```python
from build123d import *

# Parameters (mm, degrees)
SKETCH_1_W          = 15
SKETCH_1_H          = 15
SKETCH_1_W_2        = 13
SKETCH_1_H_2        = 13
EXTRUDE_1_DEPTH     = 155
SKETCH_2_R          = 1.6
CUT_EXTRUDE_1_DEPTH = 157.444878472
SKETCH_3_R          = 1.6
CUT_EXTRUDE_2_DEPTH = 157.444878472


with BuildPart() as part:
    # 草图1 → 拉伸-薄壁1 (new body)
    with BuildSketch(Plane.XY):
        with Locations((7.5, -7.5)):
            Rectangle(SKETCH_1_W, SKETCH_1_H)
        with Locations((7.5, -7.5)):
            Rectangle(SKETCH_1_W_2, SKETCH_1_H_2, mode=Mode.SUBTRACT)
    extrude(amount=EXTRUDE_1_DEPTH)

    # 草图2 → 切除-拉伸1 (cut, through all)
    with BuildSketch(Plane(origin=(15, 0, 0), x_dir=(0, 0, -1), z_dir=(1, 0, 0))):
        with Locations((-130, -3.75)):
            Circle(SKETCH_2_R)
        with Locations((-130, -11.25)):
            Circle(SKETCH_2_R)
        with Locations((-120, -11.25)):
            Circle(SKETCH_2_R)
        with Locations((-120, -3.75)):
            Circle(SKETCH_2_R)
        with Locations((-20, -3.75)):
            Circle(SKETCH_2_R)
        with Locations((-20, -11.25)):
            Circle(SKETCH_2_R)
        with Locations((-30, -11.25)):
            Circle(SKETCH_2_R)
        with Locations((-30, -3.75)):
            Circle(SKETCH_2_R)
        Polygon((-105, -1), (-110.629165125, -4.25), (-110.629165125, -10.75), (-105, -14), (-99.370834875, -10.75), (-99.370834875, -4.25), align=None)
        Polygon((-84.370834875, -10.75), (-84.370834875, -4.25), (-90, -1), (-95.629165125, -4.25), (-95.629165125, -10.75), (-90, -14), align=None)
        Polygon((-69.370834875, -10.75), (-69.370834875, -4.25), (-75, -1), (-80.629165125, -4.25), (-80.629165125, -10.75), (-75, -14), align=None)
        Polygon((-54.370834875, -10.75), (-54.370834875, -4.25), (-60, -1), (-65.629165125, -4.25), (-65.629165125, -10.75), (-60, -14), align=None)
        Polygon((-39.370834875, -10.75), (-39.370834875, -4.25), (-45, -1), (-50.629165125, -4.25), (-50.629165125, -10.75), (-45, -14), align=None)
    extrude(amount=-CUT_EXTRUDE_1_DEPTH, mode=Mode.SUBTRACT)

    # 草图3 → 切除-拉伸2 (cut, through all)
    with BuildSketch(Plane(origin=(0, 0, 0), x_dir=(1, 0, 0), z_dir=(0, 1, 0))):
        with Locations(Location((3.75, -5, 0), (0, 0, 270))):
            Circle(SKETCH_3_R)
        with Locations(Location((11.25, -5, 0), (0, 0, 90))):
            Circle(SKETCH_3_R)
        with Locations(Location((11.25, -15, 0), (0, 0, 270))):
            Circle(SKETCH_3_R)
        with Locations(Location((3.75, -15, 0), (0, 0, 90))):
            Circle(SKETCH_3_R)
        with Locations(Location((3.75, -25, 0), (0, 0, 270))):
            Circle(SKETCH_3_R)
        with Locations(Location((11.25, -25, 0), (0, 0, 90))):
            Circle(SKETCH_3_R)
        with Locations(Location((11.25, -35, 0), (0, 0, 270))):
            Circle(SKETCH_3_R)
        with Locations(Location((3.75, -35, 0), (0, 0, 90))):
            Circle(SKETCH_3_R)
        with Locations(Location((3.75, -45, 0), (0, 0, 270))):
            Circle(SKETCH_3_R)
        with Locations(Location((11.25, -45, 0), (0, 0, 90))):
            Circle(SKETCH_3_R)
        with Locations(Location((11.25, -55, 0), (0, 0, 270))):
            Circle(SKETCH_3_R)
        with Locations(Location((3.75, -55, 0), (0, 0, 90))):
            Circle(SKETCH_3_R)
        with Locations(Location((3.75, -72.5, 0), (0, 0, 270))):
            Circle(SKETCH_3_R)
        with Locations(Location((11.25, -72.5, 0), (0, 0, 90))):
            Circle(SKETCH_3_R)
        with Locations(Location((11.25, -82.5, 0), (0, 0, 270))):
            Circle(SKETCH_3_R)
        with Locations(Location((3.75, -82.5, 0), (0, 0, 90))):
            Circle(SKETCH_3_R)
        with Locations(Location((3.75, -100, 0), (0, 0, 270))):
            Circle(SKETCH_3_R)
        with Locations(Location((11.25, -100, 0), (0, 0, 90))):
            Circle(SKETCH_3_R)
        with Locations(Location((11.25, -110, 0), (0, 0, 270))):
            Circle(SKETCH_3_R)
        with Locations(Location((3.75, -110, 0), (0, 0, 90))):
            Circle(SKETCH_3_R)
        with Locations(Location((3.75, -120, 0), (0, 0, 270))):
            Circle(SKETCH_3_R)
        with Locations(Location((11.25, -120, 0), (0, 0, 90))):
            Circle(SKETCH_3_R)
        with Locations(Location((11.25, -130, 0), (0, 0, 270))):
            Circle(SKETCH_3_R)
        with Locations(Location((3.75, -130, 0), (0, 0, 90))):
            Circle(SKETCH_3_R)
        with Locations(Location((3.75, -140, 0), (0, 0, 270))):
            Circle(SKETCH_3_R)
        with Locations(Location((11.25, -140, 0), (0, 0, 90))):
            Circle(SKETCH_3_R)
        with Locations(Location((11.25, -150, 0), (0, 0, 270))):
            Circle(SKETCH_3_R)
        with Locations(Location((3.75, -150, 0), (0, 0, 90))):
            Circle(SKETCH_3_R)
    extrude(amount=-CUT_EXTRUDE_2_DEPTH, mode=Mode.SUBTRACT)


solid = part.part
```
Part model, mm, in its own coordinate system. A direction names the side the tool comes from. Round coordinates to 2 decimals unless told otherwise and drop trailing zeros. Loops run counter-clockwise (first coordinate to the right, second up) from the corner with the lowest first, then second, coordinate; pieces in that order, holes last.
Item 1: 3-axis set-ups, long thin cutter, end or side, ignore diameter. For faces 3 (the face through (1, -8, 52)), 4 (the face through (0.507, -2.648, 57.146)), 5 (the face through (12.81, -0.49, 5.35)): which of +Z, -Z, +X, -X, +Y, -Y reach the whole face in a straight line?
Item 2: Cut at D-D, the plane z = 49. Give the cut face in (x, y), then the cut area to 3 significant figures.
Item 3: Cut at C-C, the plane z = 93.5. Give the cut face in (x, y), then the cut area to 3 significant figures.
Item 4: Mould opens along Y. For faces 1 (the face through (4.231, -14.493, 121.526)), 2 (the face through (14.507, -12.352, 77.854)) say: +Y half, -Y half, draft (parallel to the pull), parting line (faces both ways), or undercut.
Item 5: Cut at B-B, the plane z = 120. State how many separate pieces and enclosed holes the cut face has, then the cut area to 3 significant figures.
Item 6: Drill centre lines: line 1 (X direction, y = -0.4, z = 5); line 2 (Y direction, x = 0.3, z = 20); line 3 (X direction, y = -11, z = 14). Where is each one in solid material? Low to high.
Item 7: Cut at A-A, the plane z = 30. Give the cut face in (x, y).
A:
1. face 3: +Z, -Z
1. face 4: +X, -X
1. face 5: +Y, -Y
2. outline: (0, -15) - (15, -15) - (15, -11.69) - (14, -11.69) - (14, -14) - (1, -14) - (1, -11.69) - (0, -11.69) - close; (0, -3.31) - (1, -3.31) - (1, -1) - (14, -1) - (14, -3.31) - (15, -3.31) - (15, 0) - (0, 0) - close
2. area: 39.2 mm2
3. outline: (0, -15) - (15, -15) - (15, -11.98) - (14, -11.98) - (14, -14) - (1, -14) - (1, -11.98) - (0, -11.98) - close; (0, -3.02) - (1, -3.02) - (1, -1) - (14, -1) - (14, -3.02) - (15, -3.02) - (15, 0) - (0, 0) - close
3. area: 38.1 mm2
4. face 1: draft
4. face 2: undercut
5. separate pieces: 8
5. enclosed holes: 0
5. area: 30.4 mm2
6. line 1: x = 0 to 2.15, 5.35 to 9.65, 12.85 to 15
6. line 2: y = -15 to -12.85, -9.65 to -5.35, -2.15 to 0
6. line 3: x = 0 to 1, 14 to 15
7. outline: (0, -15) - (15, -15) - (15, -12.85) - (14, -12.85) - (14, -14) - (1, -14) - (1, -12.85) - (0, -12.85) - close; (0, -9.65) - (1, -9.65) - (1, -5.35) - (0, -5.35) - close; (0, -2.15) - (1, -2.15) - (1, -1) - (14, -1) - (14, -2.15) - (15, -2.15) - (15, 0) - (0, 0) - close; (14, -9.65) - (15, -9.65) - (15, -5.35) - (14, -5.35) - close
